from build123d import *

# Parameters (mm, degrees)
F1_DEPTH = 102.362
F2_SIZE  = 5.08


with BuildPart() as f1:
    # F0 (on Top) → F1 (new body)
    with BuildSketch(Plane.XY):
        Polygon((17.439397, -78.062701), (79.63111, -7.536849), (31.775335, 73.404672), (-59.992873, 52.903431), (-68.85297, -40.708554), align=None)
        Polygon((14.577651, 42.818111), (45.227185, -0.632646), (13.374287, -43.209108), (-36.961421, -26.072052), (-36.217702, 27.095694), align=None, mode=Mode.SUBTRACT)
    extrude(amount=F1_DEPTH)

    # F2
    f2_edges = [f1.edges().sort_by_distance(p)[0] for p in [
        (48.535254, -42.799775, 0),
        (55.703223, 32.933912, 0),
        (-14.108769, 63.154051, 0),
        (-64.422921, 6.097439, 0),
        (-25.706786, -59.385627, 0),
        (-10.820026, 34.956902, 0),
        (29.902418, 21.092733, 0),
        (29.300736, -21.920877, 0),
        (-11.793567, -34.64058, 0),
        (-36.589562, 0.511821, 0),
        (48.535254, -42.799775, 102.362),
        (55.703223, 32.933912, 102.362),
        (-14.108769, 63.154051, 102.362),
        (-64.422921, 6.097439, 102.362),
        (-25.706786, -59.385627, 102.362),
        (-10.820026, 34.956902, 102.362),
        (29.902418, 21.092733, 102.362),
        (29.300736, -21.920877, 102.362),
        (-11.793567, -34.64058, 102.362),
        (-36.589562, 0.511821, 102.362),
    ]]
    chamfer(f2_edges, length=F2_SIZE)


solid = f1.part
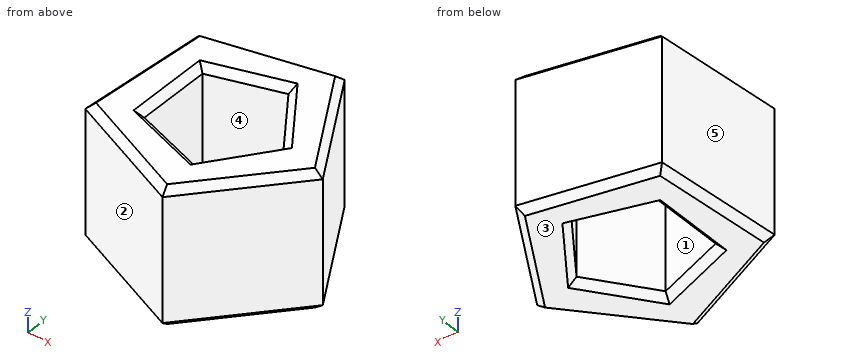
Could you check a few things on this model? Use its own coordinates, in mm. Face numbers are marked on the shaded views. A direction names the side the tool comes from. Round coordinates to 2 decimals unless told otherwise and drop trailing zeros. Write each loop counter-clockwise with the first axis right and the second up, starting at its lowest first coordinate (ties: lowest second). Pieces come first, ordered by that corner, then holes. Notation, with made-up numbers: (2, -30.5) - (18, -30.5) arc R8 ccw to (18, -24.5) - close; hole circle Ø4 at (-17.75, 37). An arc over 180 degrees is marked (long way). Use a Markdown table: item, result.
Q1. I want a section at C-C (x = -28). List the corners of the cut face in (y, z) for me, plus the area to 3 significant figures.
Output values:
| item | result |
|---|---|
| outline | (-58.39, 5.08) - (-52.86, 0) - (-34.49, 0) - (-29.12, 5.08) - (-29.12, 97.28) - (-34.49, 102.36) - (-52.86, 102.36) - (-58.39, 97.28) - close; (29.64, 5.08) - (34.96, 0) - (54.85, 0) - (60.05, 5.08) - (60.05, 97.28) - (54.85, 102.36) - (34.96, 102.36) - (29.64, 97.28) - close |
| area | 6,000 mm2 |
Q2. For pin 1 (1 mm diameter, centred on x = 7, z = 10.5, fed in from +Y); pin 2 (12 mm diameter, centred on x = 26.5, z = 30.5, fed in from -Y); pin 3 (10 mm diameter, centred on y = 10, z = 43.5, fed in from -X), each with a flat end and sliding along its axis, tell me the tip position at first contact or that it passes through.
Output values:
| item | result |
|---|---|
| pin 1 | y = 67.98 |
| pin 2 | y = -74.59 |
| pin 3 | x = -64.53 |
Q3. Please list where these lines run through material, in increasing order: L1, parallel to Y at x = 0, z = 66; L2, parallel to Y at x = 13.5, z = 51; L3, parallel to X at y = 19.5, z = 30.
Output values:
| item | result |
|---|---|
| L1 | -70.51 to -38.66, 38.31 to 66.31 |
| L2 | -76.36 to -43.04, 42.48 to 69.32 |
| L3 | -63.15 to -36.32, 31.03 to 63.65 |
Q4. I want a section at B-B (y = 9). List the corners of the cut face in (x, z) for me.
Output values:
| item | result |
|---|---|
| outline | (-64.15, 5.08) - (-59.05, 0) - (-41.55, 0) - (-36.47, 5.08) - (-36.47, 97.28) - (-41.55, 102.36) - (-59.05, 102.36) - (-64.15, 97.28) - close; (38.43, 5.08) - (44.65, 0) - (63.95, 0) - (69.85, 5.08) - (69.85, 97.28) - (63.95, 102.36) - (44.65, 102.36) - (38.43, 97.28) - close |
Q5. For the marked faces 4 and 5, which set-ups out of +Z, -Z, +X, -X, +Y, -Y let a thin tool reach every point of the face, with its end or its side?
Output values:
| item | result |
|---|---|
| face 4 | +Z, -Z |
| face 5 | +Z, -Z, -X, +Y |
Q6. I want a section at A-A (z = 49). List the corners of the cut face in (x, y) for me, plus the area to 3 significant figures.
Output values:
| item | result |
|---|---|
| outline | (-68.85, -40.71) - (17.44, -78.06) - (79.63, -7.54) - (31.78, 73.4) - (-59.99, 52.9) - close; hole (-36.96, -26.07) - (13.37, -43.21) - (45.23, -0.63) - (14.58, 42.82) - (-36.22, 27.1) - close |
| area | 10,300 mm2 |
Q7. I want a section at D-D (x = 68). List the corners of the cut face in (y, z) for me.
Output values:
| item | result |
|---|---|
| outline | (-20.73, 5.08) - (-13.05, 0) - (2.15, 0) - (12.14, 5.08) - (12.14, 97.28) - (2.15, 102.36) - (-13.05, 102.36) - (-20.73, 97.28) - close |
Q8. Thinking about a two-plate mould opening in Y: for the marked faces 1, 2 and 3, which applies, released by +Y, released by -Y, zero draft, split by the parting line, or undercut?
Output values:
| item | result |
|---|---|
| face 1 | undercut |
| face 2 | released by -Y |
| face 3 | zero draft |
